Check sheet for the modelled part. Datum: model origin and axes. Units: mm. Face numbers are marked on the shaded views. Coordinates: 2 decimals unless noted, no trailing zeros. Write each loop counter-clockwise with the first axis right and the second up, starting at its lowest first coordinate (ties: lowest second). Pieces come first, ordered by that corner, then holes. Notation, with made-up numbers: M 57,-14 L 103,-14 A16 ccw 103,12 Z; hole C -28,47.25 d9. An arc over 180 degrees is marked long. Answer as CSV lines item,"result". Start each with the question number.
1) Draft check along Z on the marked faces 1 and 2. Enter one of: +Z half, -Z half, draft (parallel to the pull), parting line (faces both ways), or undercut.
2) Material ranges on L1, parallel to Z at x = -61, y = 13.5; L2, parallel to Z at x = 12, y = 4; L3, parallel to Y at x = -2, z = 17, recorded low to high. Write a range as [from, to].
3) Section check C-C (x = -43.5). Record the cut outline in (y, z), and give its area (3 significant figures).
4) Go/stop test with flat-tipped pins: pin 1 Ø1.6 at (x, y) = (-149, 18) entering from +Z; pin 2 Ø6 at (x, z) = (-108, 31) entering from +Y; pin 3 Ø4 at (y, z) = (17.5, 87) entering from +X; pin 4 Ø3 at (x, y) = (-11.55, 14.1) entering from +Z. Record where each tip stops, or that it passes through.
5) Section check A-A (y = 10). State how many separate pieces and enclosed holes the cut face has, and give its area (3 significant figures).
6) Section check B-B (z = 35). Record the cut outline in (x, y), and give its area (3 significant figures).
from build123d import *

# Parameters (mm, degrees)
SKETCH1_W               = 175
SKETCH1_H               = 163
BOSS_EXTRUDE1_DEPTH     = 5
SKETCH2_W               = 20
SKETCH2_H               = 5
BOSS_EXTRUDE2_DEPTH     = 18
SKETCH3_R               = 2
CUT_EXTRUDE1_DEPTH      = 7
CUT_EXTRUDE1_DEPTH_BACK = 158
SKETCH4_W               = 5.5
SKETCH4_H               = 15
SKETCH4_W_2             = 6
SKETCH4_H_2             = 10
BOSS_EXTRUDE3_DEPTH     = 18
SKETCH5_R               = 2
CUT_EXTRUDE2_DEPTH      = 18
SKETCH6_W               = 5.5
SKETCH6_H               = 15
BOSS_EXTRUDE4_DEPTH     = 10
SKETCH7_R               = 2
CUT_EXTRUDE3_DEPTH      = 10
SKETCH8_W               = 4.2
SKETCH8_H               = 8
CUT_EXTRUDE4_DEPTH      = 10
SKETCH9_R               = 2
CUT_EXTRUDE5_DEPTH      = 18


with BuildPart() as part:
    # Sketch1 → Boss-Extrude1 (new body)
    with BuildSketch(Plane(origin=(0, 0, 0), x_dir=(1, 0, 0), z_dir=(0, 1, 0))):
        with Locations((-64.046391753, -12.943298969)):
            Rectangle(SKETCH1_W, SKETCH1_H)
    extrude(amount=BOSS_EXTRUDE1_DEPTH)

    # Sketch2 → Boss-Extrude2 (add)
    with BuildSketch(Plane(origin=(0, 5, 0), x_dir=(1, 0, 0), z_dir=(0, 1, 0))):
        with Locations((-116.546391753, 66.056701031)):
            Rectangle(SKETCH2_W, SKETCH2_H)
        with Locations((-116.546391753, -85.943298969)):
            Rectangle(SKETCH2_W, SKETCH2_H)
        with Locations((-11.546391753, -85.943298969)):
            Rectangle(SKETCH2_W, SKETCH2_H)
        with Locations((-11.546391753, 66.056701031)):
            Rectangle(SKETCH2_W, SKETCH2_H)
        with Locations((-64.046391753, -85.943298969)):
            Rectangle(SKETCH2_W, SKETCH2_H)
        with Locations((-64.046391753, 66.056701031)):
            Rectangle(SKETCH2_W, SKETCH2_H)
    extrude(amount=BOSS_EXTRUDE2_DEPTH)

    # Sketch3 → Cut-Extrude1 (cut, two sides)
    with BuildSketch(Plane.XY.offset(88.443298969)) as cut_extrude1_sk:
        with Locations((-116.546391753, 14.1)):
            Circle(SKETCH3_R)
        with Locations((-64.046391753, 14.1)):
            Circle(SKETCH3_R)
        with Locations((-11.546391753, 14.1)):
            Circle(SKETCH3_R)
    extrude(amount=CUT_EXTRUDE1_DEPTH, mode=Mode.SUBTRACT)
    extrude(cut_extrude1_sk.sketch, amount=-CUT_EXTRUDE1_DEPTH_BACK, mode=Mode.SUBTRACT)

    # Sketch4 → Boss-Extrude3 (add)
    with BuildSketch(Plane(origin=(0, 5, 0), x_dir=(1, 0, 0), z_dir=(0, 1, 0))):
        with Locations((-148.796391753, 61.056701031)):
            Rectangle(SKETCH4_W, SKETCH4_H)
        with Locations((-148.546391753, -83.443298969)):
            Rectangle(SKETCH4_W_2, SKETCH4_H_2)
    extrude(amount=BOSS_EXTRUDE3_DEPTH)

    # Sketch5 → Cut-Extrude2 (cut)
    with BuildSketch(Plane(origin=(-146.046391753, 0, 0), x_dir=(0, 0, -1), z_dir=(1, 0, 0))):
        with Locations((64.556701031, 14.1)):
            Circle(SKETCH5_R)
    extrude(amount=-CUT_EXTRUDE2_DEPTH, mode=Mode.SUBTRACT)

    # Sketch6 → Boss-Extrude4 (add)
    with BuildSketch(Plane(origin=(0, 5, 0), x_dir=(1, 0, 0), z_dir=(0, 1, 0))):
        with Locations((20.703608247, 61.056701031)):
            Rectangle(SKETCH6_W, SKETCH6_H)
    extrude(amount=BOSS_EXTRUDE4_DEPTH)

    # Sketch7 → Cut-Extrude3 (cut)
    with BuildSketch(Plane(origin=(23.453608247, 0, 0), x_dir=(0, 0, -1), z_dir=(1, 0, 0))):
        with Locations((61.056701031, 10)):
            Circle(SKETCH7_R)
    extrude(amount=-CUT_EXTRUDE3_DEPTH, mode=Mode.SUBTRACT)

    # Sketch8 → Cut-Extrude4 (cut)
    with BuildSketch(Plane(origin=(0, 5, 0), x_dir=(1, 0, 0), z_dir=(0, 1, 0))):
        with Locations((16.353608247, -60.443298969)):
            Rectangle(SKETCH8_W, SKETCH8_H)
        with Locations((16.353608247, -22.443298969)):
            Rectangle(SKETCH8_W, SKETCH8_H)
        with Locations((16.353608247, 15.556701031)):
            Rectangle(SKETCH8_W, SKETCH8_H)
    extrude(amount=-CUT_EXTRUDE4_DEPTH, mode=Mode.SUBTRACT)

    # Sketch9 → Cut-Extrude5 (cut)
    with BuildSketch(Plane(origin=(23.453608247, 0, 0), x_dir=(0, 0, -1), z_dir=(1, 0, 0))):
        with Locations((-60.443298969, 2.5)):
            Circle(SKETCH9_R)
        with Locations((15.556701031, 2.5)):
            Circle(SKETCH9_R)
        with Locations((-22.443298969, 2.5)):
            Circle(SKETCH9_R)
    extrude(amount=-CUT_EXTRUDE5_DEPTH, mode=Mode.SUBTRACT)


solid = part.part
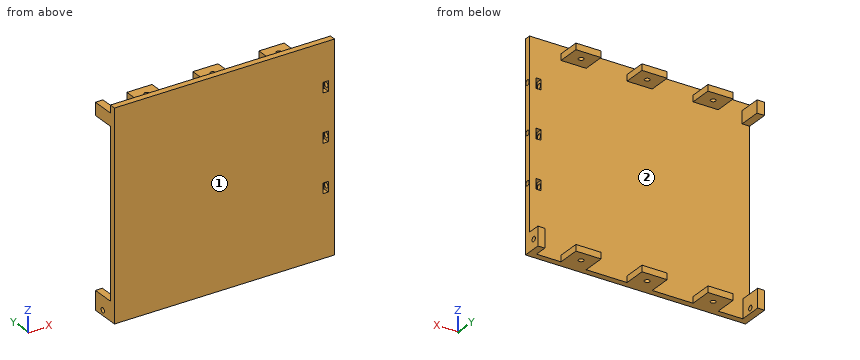
Results found:
1,face 1,"draft"
1,face 2,"undercut"
2,L1,"z = [-68.56, -63.56], [83.44, 88.44]"
2,L2,"z = [-68.56, -16.88], [-14.23, 21.12], [23.77, 59.12], [61.77, 94.44]"
2,L3,"y = [0, 5]"
3,outline,"M 0,-68.56 L 5,-68.56 L 5,94.44 L 0,94.44 Z"
3,area,"815 mm2"
4,pin 1,"stops at z = 88.44"
4,pin 2,"stops at y = 5"
4,pin 3,"stops at x = -1.55"
4,pin 4,"passes through"
5,separate pieces,"10"
5,enclosed holes,"0"
5,area,"803 mm2"
6,outline,"M -151.55,0 L 23.45,0 L 23.45,5 L -151.55,5 Z"
6,area,"875 mm2"
